Check sheet for the modelled part. Datum: model origin and axes. Units: mm. A direction names the side the tool comes from. Round coordinates to 2 decimals unless told otherwise and drop trailing zeros. Order: outer loops, then holes, each group sorted by start corner. A loop starts at its lowest first (then second) coordinate and runs counter-clockwise, first axis right, second up.
Q1. Mould release check, pull along X, two halves, no side actions. Record for faces 5 (the flat face through (0, 14.75, -6)), 6 (the flat face through (-7.2, 14.75, -15.4)), 7 (the flat face through (4.542, 0.616, 4.603)): +X half, -X half, draft (parallel to the pull), parting line (faces both ways), or undercut.
Q2. Scan lines: probe 1 along Y at (x, z) = (2, -10); probe 2 along X at (y, z) = (11.5, -1.5); probe 3 along Z at (x, y) = (31, 5.5). Record each from-to range of solid material in increasing order.
Q3. Set-up check for faces 1 (the flat face through (-35, 8, 0)), 2 (the flat face through (32, 8, 1.25)), 3 (the flat face through (9.85, 7.91, -9.73)), 4 (the flat face through (-31, 8, 1.25)): record each of +Z, -Z, +X, -X, +Y, -Y from which the full face is reachable in a straight line by a thin tool's end or side.
Q4. Cross-section at D-D on z = -17.5. Record the cut outline in (x, y), then the cut area to 3 significant figures.
Q5. Cross-section at A-A on z = -6. Record the cut outline in (x, y), then the cut area to 3 significant figures.
Q6. Cross-section at C-C on x = 37. Record the cut outline in (y, z).
Q7. Depth check by flat-ended pin: P1, Ø8, axis at x = 18.5, y = 9, coming from the +Z side; P2, Ø1.5, axis at x = -7.5, y = 13, coming from the +Z side; P3, Ø3, axis at y = 7.5, z = -5, coming from the -X side. Enter the tip coordinate at first touch or a pass-through.
from build123d import *

# Parameters (mm, degrees)
BOSS_EXTRUDE1_DEPTH  = 1.25
BOSS_EXTRUDE8_START  = -8
BOSS_EXTRUDE8_DEPTH  = 16
CHAMFER2_SIZE2       = 3
CHAMFER2_SIZE        = 1.25
CHAMFER3_SIZE2       = 3
CHAMFER3_SIZE        = 1.25
BOSS_EXTRUDE9_DEPTH  = 1.25
BOSS_EXTRUDE10_DEPTH = 1.25
CUT_EXTRUDE1_REACH   = 59.082
SKETCH6_R            = 0.5


with BuildPart() as part:
    # Sketch1 → Boss-Extrude1 (new body)
    with BuildSketch(Plane(origin=(0, 0, 0), x_dir=(1, 0, 0), z_dir=(0, 1, 0))):
        with BuildLine():
            Line((-50, 0), (-2.082988952, 21.95833302))
            ThreePointArc((-2.082988952, 21.95833302), (0, 22.412878475), (2.082988952, 21.95833302))
            Line((2.082988952, 21.95833302), (50, 0))
            Line((50, 0), (20, 0))
            Line((20, 0), (0.753370804, 22.049783791))
            ThreePointArc((0.753370804, 22.049783791), (0, 22.392187842), (-0.753370804, 22.049783791))
            Line((-0.753370804, 22.049783791), (-20, 0))
            Line((-20, 0), (-50, 0))
        make_face()
    extrude(amount=BOSS_EXTRUDE1_DEPTH)


with BuildPart() as body_2:
    # Body-Move/Copy1: copy of part
    add(part.part.moved(Location((0, 14.75, 0))))


with BuildPart() as part_1:
    add(part.part)

    add(body_2.part)  # Boss-Extrude8 merges body 2
    # Sketch3 → Boss-Extrude8 (add)
    with BuildSketch(Plane(origin=(0, 8, 0), x_dir=(1, 0, 0), z_dir=(0, 1, 0)).offset(BOSS_EXTRUDE8_START)):
        with BuildLine():
            Line((19.431879943, -1.25), (0, 21.012015184))
            Line((0, 21.012015184), (-19.431879943, -1.25))
            Line((-19.431879943, -1.25), (-50, -1.25))
            Line((-50, -1.25), (-50, 0))
            Line((-50, 0), (-20, 0))
            Line((-20, 0), (-0.753370804, 22.049783791))
            ThreePointArc((-0.753370804, 22.049783791), (0, 22.392187842), (0.753370804, 22.049783791))
            Line((0.753370804, 22.049783791), (20, 0))
            Line((20, 0), (50, 0))
            Line((50, 0), (50, -1.25))
            Line((50, -1.25), (19.431879943, -1.25))
        make_face()
    extrude(amount=BOSS_EXTRUDE8_DEPTH)

    # Chamfer2
    chamfer2_edges = [part_1.edges().sort_by_distance(p)[0] for p in [
        (50, 8, 1.25),
    ]]
    chamfer2_side = [part_1.faces().sort_by_distance(p)[0] for p in [
        (50, 8, 1.225),
    ]]
    chamfer(chamfer2_edges, length=CHAMFER2_SIZE - 0.0001, length2=CHAMFER2_SIZE2 - 0.0001, reference=chamfer2_side[0])  # a hair under: the kernel refuses the full size

    # Chamfer3
    chamfer3_edges = [part_1.edges().sort_by_distance(p)[0] for p in [
        (-50, 8, 1.25),
    ]]
    chamfer3_side = [part_1.faces().sort_by_distance(p)[0] for p in [
        (-50, 8, 1.225),
    ]]
    chamfer(chamfer3_edges, length=CHAMFER3_SIZE - 0.0001, length2=CHAMFER3_SIZE2 - 0.0001, reference=chamfer3_side[0])  # a hair under: the kernel refuses the full size

    # Sketch4 → Boss-Extrude9 (add)
    with BuildSketch(Plane(origin=(0, 16, 0), x_dir=(1, 0, 0), z_dir=(0, 1, 0))):
        Polygon((-19.431879943, -1.25), (0, 21.012015184), (19.431879943, -1.25), align=None)
    boss_extrude9 = extrude(amount=-BOSS_EXTRUDE9_DEPTH)

    # Mirror1: Boss-Extrude9 across plane
    add(boss_extrude9.mirror(Plane.ZX.offset(8)))

    # Sketch5 → Boss-Extrude10 (add)
    with BuildSketch(Plane.XZ):
        with BuildLine():
            Line((-7.5, 1.25), (7.5, 1.25))
            Line((7.5, 1.25), (1.499675711, 8.050367528))
            ThreePointArc((1.499675711, 8.050367528), (0, 8.727124254), (-1.499675711, 8.050367528))
            Line((-1.499675711, 8.050367528), (-7.5, 1.25))
        make_face()
    boss_extrude10 = extrude(amount=-BOSS_EXTRUDE10_DEPTH)

    # Mirror2: Boss-Extrude10 across plane
    add(boss_extrude10.mirror(Plane.ZX.offset(8)))

    # Sketch6 → Cut-Extrude1 (cut, up to next)
    with BuildSketch(Plane(origin=(0, 0, 0), x_dir=(-1, 0, 0), z_dir=(0, -1, 0)), mode=Mode.PRIVATE) as cut_extrude1_sk1:
        with Locations(Location((0, -5.727124254, 0), (0, 0, 90))):
            Circle(SKETCH6_R)
    cut_extrude1_tool1 = extrude(cut_extrude1_sk1.sketch, amount=-CUT_EXTRUDE1_REACH, mode=Mode.PRIVATE) & part_1.part
    add(cut_extrude1_tool1.solids().sort_by_distance((0, 0, 5.727124))[0], mode=Mode.SUBTRACT)
    add(cut_extrude1_tool1.solids().sort_by_distance((0, 0, 5.727124))[1], mode=Mode.SUBTRACT)


solid = part_1.part
Results found:
1. face 5: undercut
1. face 6: draft
1. face 7: +X half
2. probe 1: y = 0 to 1.25, 14.75 to 16
2. probe 2: x = -18.69 to -17.03, 17.03 to 18.69
2. probe 3: z = 0 to 1.25
3. face 1: -Z, -X
3. face 2: +Z, +X, +Y, -Y
3. face 3: +Z
3. face 4: +Z, -X, +Y, -Y
4. outline: (-11.81, 0) - (11.81, 0) - (11.81, 1.25) - (4.72, 1.25) - (4.72, 14.75) - (11.81, 14.75) - (11.81, 16) - (-11.81, 16) - (-11.81, 14.75) - (-4.72, 14.75) - (-4.72, 1.25) - (-11.81, 1.25) - close; hole (-3.07, 1.25) - (3.07, 1.25) - (3.07, 14.75) - (-3.07, 14.75) - close
4. area: 104 mm2
5. outline: (-36.91, 0) - (36.91, 0) - (36.91, 1.25) - (14.76, 1.25) - (14.76, 14.75) - (36.91, 14.75) - (36.91, 16) - (-36.91, 16) - (-36.91, 14.75) - (-14.76, 14.75) - (-14.76, 1.25) - (-36.91, 1.25) - close; hole (-13.1, 1.25) - (13.1, 1.25) - (13.1, 14.75) - (-13.1, 14.75) - close
5. area: 229 mm2
6. outline: (0, -5.96) - (1.25, -5.96) - (1.25, 0) - (14.75, 0) - (14.75, -5.96) - (16, -5.96) - (16, 1.25) - (0, 1.25) - close
7. P1: stops at z = 1.25
7. P2: stops at z = -11.56
7. P3: stops at x = -16.94
